Work out the finished part from the listing and answer in its coordinate system (mm). A direction names the side the tool comes from. Give positions to 0.01 mm unless a question says otherwise; leave off trailing zeros. Loops run counter-clockwise (first coordinate to the right, second up) from the corner with the lowest first, then second, coordinate; pieces in that order, holes last. Notation, with made-up numbers: (35, -30) - (58, -30) arc R29 ccw to (58, -5) - close; hole circle Ø5 at (51, 11.25). An arc over 180 degrees is marked (long way). One line per item, written item: value.
from build123d import *

# Parameters (mm, degrees)
F1_DEPTH = 5
F4_SIZE  = 2
F5_R     = 5
F6_R     = 5
F8_DEPTH = 0.5


with BuildPart() as f1:
    # F0 (on Top) → F1 (new body, symmetric)
    with BuildSketch(Plane.XY):
        with BuildLine():
            ThreePointArc((9.9498743711, -1), (-0.5006277506, -9.9874607311), (-10, 0))
            Line((-10, 0), (-10, 1.5))
            Line((-10, 1.5), (-11, 1.5))
            Line((-11, 1.5), (-13, -2.5))
            Line((-13, -2.5), (-11, -2.5))
            Line((-11, -2.5), (-11, -12))
            Line((-11, -12), (12, -12))
            Line((12, -12), (12, 11))
            Line((12, 11), (-14.8090169944, 11))
            Line((-14.8090169944, 11), (-14.8090169944, -11))
            Line((-14.8090169944, -11), (-11.5, -11))
            Line((-11.5, -11), (-11.5, -3))
            Line((-11.5, -3), (-13.8090169944, -3))
            Line((-13.8090169944, -3), (-11.3090169944, 2))
            Line((-11.3090169944, 2), (-9.7979589711, 2))
            ThreePointArc((-9.7979589711, 2), (0.5057366629, 9.9872033337), (9.9498743711, 1))
            Line((9.9498743711, 1), (11, 1))
            Line((11, 1), (11, -1))
            Line((11, -1), (9.9498743711, -1))
        make_face()
    extrude(amount=F1_DEPTH, both=True)

    # F2 (on Top) → F3 (revolve, cut)
    with BuildSketch(Plane.XY):
        Polygon((0, 0), (-10, 0), (-10, -3.5), (-2, -11.5), (-2, -12), (0, -12), align=None)
    revolve(axis=Axis((0, -5.25, 0), (0, -1, 0)), mode=Mode.SUBTRACT)

    # F4
    f4_edges = [f1.edges().sort_by_distance(p)[0] for p in [
        (-11.5, -11, 0),
    ]]
    chamfer(f4_edges, length=F4_SIZE)

    # F5
    f5_edges = [f1.edges().sort_by_distance(p)[0] for p in [
        (12, 11, 0),
    ]]
    fillet(f5_edges, radius=F5_R)

    # F6
    f6_edges = [f1.edges().sort_by_distance(p)[0] for p in [
        (-14.809017, 11, 0),
    ]]
    fillet(f6_edges, radius=F6_R)

    # F7 (on face) → F8 (join)
    with BuildSketch(Plane(origin=(0, 11, 0), x_dir=(-1, 0, 0), z_dir=(0, 1, 0))):
        with BuildLine():
            add(Edge.make_bspline(
                [(4.1006944444, -2.24609375), (4.1006944444, -3.5894097222), (3.1338975694, -4.3630642361)],
                knots=[0, 0, 0, 1, 1, 1], degree=2))
            add(Edge.make_bspline(
                [(3.5852864583, -0.6087239583), (4.1006944444, -1.2760416667), (4.1006944444, -2.24609375)],
                knots=[0, 0, 0, 1, 1, 1], degree=2))
            add(Edge.make_bspline(
                [(1.6788194444, 0.7248263889), (3.0698784722, 0.05859375), (3.5852864583, -0.6087239583)],
                knots=[0, 0, 0, 1, 1, 1], degree=2))
            add(Edge.make_bspline(
                [(0.3474392361, 1.4192708333), (0.6284722222, 1.2261284722), (1.6788194444, 0.7248263889)],
                knots=[0, 0, 0, 1, 1, 1], degree=2))
            add(Edge.make_bspline(
                [(-0.0627170139, 1.8196614583), (0.06640625, 1.6124131944), (0.3474392361, 1.4192708333)],
                knots=[0, 0, 0, 1, 1, 1], degree=2))
            add(Edge.make_bspline(
                [(-0.1918402778, 2.3046875), (-0.1918402778, 2.0269097222), (-0.0627170139, 1.8196614583)],
                knots=[0, 0, 0, 1, 1, 1], degree=2))
            add(Edge.make_bspline(
                [(0.1271701389, 3.0295138889), (-0.1918402778, 2.7517361111), (-0.1918402778, 2.3046875)],
                knots=[0, 0, 0, 1, 1, 1], degree=2))
            add(Edge.make_bspline(
                [(1.04296875, 3.3072916667), (0.4461805556, 3.3072916667), (0.1271701389, 3.0295138889)],
                knots=[0, 0, 0, 1, 1, 1], degree=2))
            add(Edge.make_bspline(
                [(2.0629340278, 3.1781684028), (1.5442708333, 3.3072916667), (1.04296875, 3.3072916667)],
                knots=[0, 0, 0, 1, 1, 1], degree=2))
            add(Edge.make_bspline(
                [(3.3758680556, 2.7235243056), (2.5815972222, 3.0490451389), (2.0629340278, 3.1781684028)],
                knots=[0, 0, 0, 1, 1, 1], degree=2))
            Line((3.3758680556, 2.7235243056), (4.0529513889, 4.3598090278))
            add(Edge.make_bspline(
                [(2.5848524306, 4.8741319444), (3.2868923611, 4.6918402778), (4.0529513889, 4.3598090278)],
                knots=[0, 0, 0, 1, 1, 1], degree=2))
            add(Edge.make_bspline(
                [(1.9480484116, 5), (2.2733914608, 4.9550058902), (2.5848524306, 4.8741319444)],
                knots=[0.5563486403, 0.5563486403, 0.5563486403, 1, 1, 1], degree=2))
            Line((1.9480484116, 5), (0.2994075141, 5))
            add(Edge.make_bspline(
                [(-1.3550347222, 4.3044704861), (-0.707430669, 4.8504432463), (0.2994075141, 5)],
                knots=[0, 0, 0, 0.7260728655, 0.7260728655, 0.7260728655], degree=2))
            add(Edge.make_bspline(
                [(-2.2469618056, 2.2352430556), (-2.2469618056, 3.5525173611), (-1.3550347222, 4.3044704861)],
                knots=[0, 0, 0, 1, 1, 1], degree=2))
            add(Edge.make_bspline(
                [(-1.9756944444, 1.015625), (-2.2469618056, 1.5386284722), (-2.2469618056, 2.2352430556)],
                knots=[0, 0, 0, 1, 1, 1], degree=2))
            add(Edge.make_bspline(
                [(-1.2497829861, 0.0998263889), (-1.7044270833, 0.4926215278), (-1.9756944444, 1.015625)],
                knots=[0, 0, 0, 1, 1, 1], degree=2))
            add(Edge.make_bspline(
                [(0.1119791667, -0.7204861111), (-0.7951388889, -0.29296875), (-1.2497829861, 0.0998263889)],
                knots=[0, 0, 0, 1, 1, 1], degree=2))
            add(Edge.make_bspline(
                [(1.3977864583, -1.3921440972), (1.08203125, -1.1827256944), (0.1119791667, -0.7204861111)],
                knots=[0, 0, 0, 1, 1, 1], degree=2))
            add(Edge.make_bspline(
                [(1.8763020833, -1.8294270833), (1.7135416667, -1.6015625), (1.3977864583, -1.3921440972)],
                knots=[0, 0, 0, 1, 1, 1], degree=2))
            add(Edge.make_bspline(
                [(2.0390625, -2.3480902778), (2.0390625, -2.0572916667), (1.8763020833, -1.8294270833)],
                knots=[0, 0, 0, 1, 1, 1], degree=2))
            add(Edge.make_bspline(
                [(1.6690538194, -3.134765625), (2.0390625, -2.87109375), (2.0390625, -2.3480902778)],
                knots=[0, 0, 0, 1, 1, 1], degree=2))
            add(Edge.make_bspline(
                [(0.6089409722, -3.3984375), (1.2990451389, -3.3984375), (1.6690538194, -3.134765625)],
                knots=[0, 0, 0, 1, 1, 1], degree=2))
            add(Edge.make_bspline(
                [(-0.6638454861, -3.2161458333), (0.0316840278, -3.3984375), (0.6089409722, -3.3984375)],
                knots=[0, 0, 0, 1, 1, 1], degree=2))
            add(Edge.make_bspline(
                [(-2.3619791667, -2.5846354167), (-1.359375, -3.0338541667), (-0.6638454861, -3.2161458333)],
                knots=[0, 0, 0, 1, 1, 1], degree=2))
            Line((-2.3619791667, -2.5846354167), (-2.3619791667, -4.5377604167))
            add(Edge.make_bspline(
                [(-0.987512741, -5), (-1.7250538132, -4.8505564977), (-2.3619791667, -4.5377604167)],
                knots=[0.477766543, 0.477766543, 0.477766543, 1, 1, 1], degree=2))
            Line((-0.987512741, -5), (1.7597890221, -5))
            add(Edge.make_bspline(
                [(3.1338975694, -4.3630642361), (2.5735213253, -4.8114910174), (1.7597890221, -5)],
                knots=[0, 0, 0, 0.5796214889, 0.5796214889, 0.5796214889], degree=2))
        make_face()
    extrude(amount=F8_DEPTH)


solid = f1.part
1. For faces 1 (the conical face through (-9.4, -4.1, 0)), 2 (the flat face through (-11, -7, 0)), 3 (the flat face through (11, 0, 0)), determine the directions among +Z, -Z, +X, -X, +Y, -Y from which every point of the face is accessible in a straight line to the end or side of a thin tool.
Output:
face 1: none
face 2: +Z, -Z, -Y
face 3: +Z, -Z
2. Find the intervals of material crossed by line 1 along X through (y, z) = (-11.55, 0); line 2 along X through (y, z) = (-9, -4); line 3 along Y through (x, z) = (-12.25, 1.25), in increasing order.
Output:
line 1: x = -11 to -2, 2 to 12
line 2: x = -14.81 to -11.5, -11 to -4.36, 4.36 to 12
line 3: y = -9.75 to -3, -2.5 to -1, 0.12 to 10.36
3. Section A-A (y = -4) is taken. Write down the section's boundary in (x, z), and give its area (3 significant figures).
Output:
outline: (-14.81, -5) - (-11.5, -5) - (-11.5, 5) - (-14.81, 5) - close; (-11, -5) - (-9.17, -5) - (-9.17, -2.5) arc R9.5 cw to (-9.17, 2.5) - (-9.17, 5) - (-11, 5) - close; (9.17, -5) - (12, -5) - (12, 5) - (9.17, 5) - (9.17, 2.5) arc R9.5 cw to (9.17, -2.5) - close
area: 77.5 mm²
4. Flat-ended cylindrical pins translate along their axes: pin 1 Ø2.5 at (x, z) = (-12.5, -1.5) entering from +Y; pin 2 Ø4 at (y, z) = (8.5, -3.5) entering from +X; pin 3 Ø3 at (x, z) = (-6, 0.5) entering from +Y. Find the tip coordinate at first contact, or state that the pin passes through.
Output:
pin 1: stops at y = 10.79
pin 2: stops at x = 11.97
pin 3: stops at y = 11
5. The mould has two halves that part along Y. Classify faces 4 (the flat face through (-14.809, -2, 0)), 5 (the flat face through (-12, -2.5, 0)), 6 (the cylindrical face through (-13.31, 9.57, 0.07)): released by +Y, released by -Y, zero draft, split by the parting line, or undercut.
Output:
face 4: zero draft
face 5: undercut
face 6: released by +Y
6. Section B-B (y = 7.25) is taken. Write down the section's boundary in (x, z), and give its area (3 significant figures).
Output:
outline: (-14.65, -5) - (-6.89, -5) - (-6.89, 5) - (-14.65, 5) - close; (6.89, -5) - (11.84, -5) - (11.84, 5) - (6.89, 5) - close
area: 127 mm²
7. Section C-C (y = 0.5) is taken. Write down the section's boundary in (x, z), and give its area (3 significant figures).
Output:
outline: (-14.81, -5) - (-12.06, -5) - (-12.06, 5) - (-14.81, 5) - close; (-11.5, -5) - (-10, -5) - (-10, 5) - (-11.5, 5) - close; (11, -5) - (12, -5) - (12, 5) - (11, 5) - close
area: 52.5 mm²
